Verification items for the finished model (mm, model axes). Face numbers are marked on the shaded views. Round coordinates to 2 decimals unless told otherwise and drop trailing zeros. Loops run counter-clockwise (first coordinate to the right, second up) from the corner with the lowest first, then second, coordinate; pieces in that order, holes last.
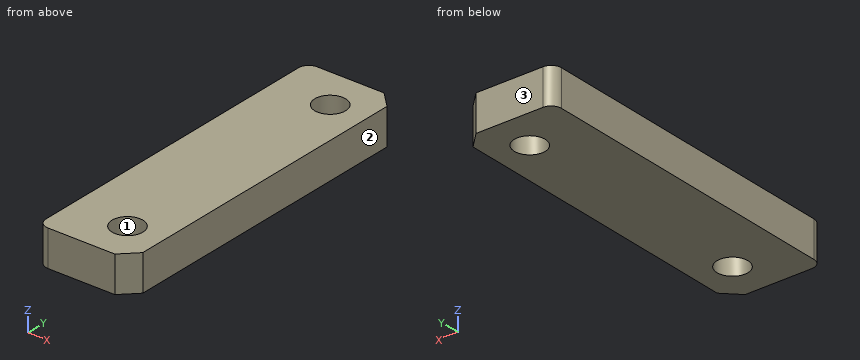
Autodesk Inventor part; units mm, degrees
ref_plane "YZ Plane" through (0, 0, 0) normal (1, 0, 0) x (0, 1, 0)
ref_plane "XZ Plane" through (0, 0, 0) normal (0, 1, 0) x (-1, 0, 0)
ref_plane "XY Plane" through (0, 0, 0) normal (0, 0, 1) x (1, 0, 0)
sketch "Szkic1" plane through (0, 0, 0) normal (0, 0, 1) x (1, 0, 0)
  circle A0 centre (9.199, -9.5538) radius 1.5
  circle A1 centre (9.199, 14.8462) radius 1.5
  line L0 (-3.801, -13.5538) -> (-5.301, -12.0538)
  line L1 (-3.801, -13.5538) -> (11.199, -13.5538)
  line L2 (12.699, -12.0538) -> (11.199, -13.5538)
  line L3 (12.699, 17.3462) -> (12.699, -12.0538)
  line L4 (11.199, 18.8462) -> (12.699, 17.3462)
  line L5 (11.199, 18.8462) -> (-3.801, 18.8462)
  line L6 (-5.301, 17.3462) -> (-3.801, 18.8462)
  line L7 (-5.301, 17.3462) -> (-5.301, -12.0538)
  circle A2 centre (0.699, -7.3538) radius 1.5
  circle A3 centre (0.699, 12.6462) radius 1.5
  line L8 (3.699, 18.8462) -> (3.699, -13.5538)
  point P0 (0, 0)
  point P1 (0, 0)
  dimension "d0" = 9
extrude "Wyciągnięcie proste1" add sketch "Szkic1" along normal blind 3.5 contours L8 L5 L4 L3 L2 L1
fillet "Zaokrąglenie1" radius 1 2 edges at (3.699, -13.5538, 1.75) (3.699, 18.8462, 1.75)
properties part number "3DP_ABS_E3D_Titan_Mounting_Plate_Spacer"
1. Gauge pin test, flat end, axial feed: P1, Ø2.5, axis at x = 9.2, y = 14.85, coming from the +Z side. Record the tip position at first contact, or that the pin passes through.
2. Section check A-A (y = -10). Enter the section's corners in (x, z).
3. Release check for a two-part mould opening along Y. For the marked faces 1, 2 and 3 record: released by +Y, released by -Y, zero draft, split by the parting line, or undercut.
4. Section check B-B (z = 2.2). Enter the section's corners in (x, y), then the cut area to 3 significant figures.
5. Section check C-C (x = 9.25). Enter the section's corners in (y, z).
6. Scan lines: L1, parallel to X at y = -9.5, z = 1.95; L2, parallel to Y at x = 9, z = 0.4; L3, parallel to Y at x = 8.25, z = 2.2. Record each from-to range of solid material in increasing order.
Taken from the geometry:
1. P1: passes through
2. outline: (3.7, 0) - (7.77, 0) - (7.77, 3.5) - (3.7, 3.5) - close; (10.63, 0) - (12.7, 0) - (12.7, 3.5) - (10.63, 3.5) - close
3. face 1: undercut
3. face 2: zero draft
3. face 3: released by +Y
4. outline: (3.7, -12.55) arc R1 ccw to (4.7, -13.55) - (11.2, -13.55) - (12.7, -12.05) - (12.7, 17.35) - (11.2, 18.85) - (4.7, 18.85) arc R1 ccw to (3.7, 17.85) - close; hole circle Ø3 at (9.2, -9.55); hole circle Ø3 at (9.2, 14.85)
4. area: 275 mm2
5. outline: (-13.55, 0) - (-11.05, 0) - (-11.05, 3.5) - (-13.55, 3.5) - close; (-8.05, 0) - (13.35, 0) - (13.35, 3.5) - (-8.05, 3.5) - close; (16.35, 0) - (18.85, 0) - (18.85, 3.5) - (16.35, 3.5) - close
6. L1: x = 3.7 to 7.7, 10.7 to 12.7
6. L2: y = -13.55 to -11.04, -8.07 to 13.36, 16.33 to 18.85
6. L3: y = -13.55 to -10.72, -8.39 to 13.68, 16.01 to 18.85
